```python
from build123d import *

# Parameters (mm, degrees)
F1_DEPTH  = 7.5
F2_DEPTH  = 1.5
F3_DEPTH  = 2
F5_DEPTH  = 45
F6_DEPTH  = 45
F7_W      = 9.5182569801
F7_H      = 1
F8_DEPTH  = 0.5
F9_W      = 12.8092049275
F9_H      = 1
F10_DEPTH = 0.5
F11_R     = 0.49999
F12_R     = 0.49999
F13_W     = 30
F13_H     = 7.6395883262
F14_DEPTH = 11.5
F16_DEPTH = 12.5


# Not quite as in the source:
# - a fillet or chamfer is up to 0.001 mm smaller than in the source, because OpenCascade refuses the exact size


with BuildPart() as f1:
    # F0 (on Front) → F1 (new body)
    with BuildSketch(Plane.XZ):
        with BuildLine():
            Line((-20.75, -40.25), (20.75, -40.25))
            Line((20.75, -40.25), (20.75, -22.75))
            Line((20.75, -22.75), (-9.25, -22.75))
            Line((-9.25, -22.75), (-9.25, 5.25))
            Line((-9.25, 5.25), (20.75, 5.25))
            Line((20.75, 5.25), (20.75, 40.25))
            Line((20.75, 40.25), (-20.75, 40.25))
            Line((-20.75, 40.25), (-20.75, 12.4785664195))
            Line((-20.75, 12.4785664195), (-12.9531003366, 17.9380143384))
            ThreePointArc((-12.9531003366, 17.9380143384), (-2.707082866, 36.9857818255), (14, 23.25))
            ThreePointArc((14, 23.25), (5.1184768061, 10.2192212364), (-10.2573135979, 13.7217515905))
            Line((-10.2573135979, 13.7217515905), (-20.75, 6.3746934757))
            Line((-20.75, 6.3746934757), (-20.75, -40.25))
        make_face()
    extrude(amount=F1_DEPTH)

    # F0 (on Front) → F2 (join)
    with BuildSketch(Plane.XZ):
        with BuildLine():
            ThreePointArc((-12.9531003366, 17.9380143384), (-11.7951280893, 15.7084515279), (-10.2573135979, 13.7217515905))
            Line((-10.2573135979, 13.7217515905), (-6.7277993643, 16.1931440631))
            ThreePointArc((-6.7277993643, 16.1931440631), (-8.3148780488, 18.158310395), (-9.3438531565, 20.4652364212))
            Line((-9.3438531565, 20.4652364212), (-12.9531003366, 17.9380143384))
        make_face()
        with BuildLine():
            Line((-6.7277993643, 16.1931440631), (-10.2573135979, 13.7217515905))
            ThreePointArc((-10.2573135979, 13.7217515905), (5.1184768061, 10.2192212364), (14, 23.25))
            ThreePointArc((14, 23.25), (-2.707082866, 36.9857818255), (-12.9531003366, 17.9380143384))
            Line((-12.9531003366, 17.9380143384), (-9.3438531565, 20.4652364212))
            ThreePointArc((-9.3438531565, 20.4652364212), (-1.4071125975, 32.8979290077), (9.75, 23.25))
            ThreePointArc((9.75, 23.25), (3.8383887374, 14.2873401325), (-6.7277993643, 16.1931440631))
        make_face()
    extrude(amount=F2_DEPTH)

    # F0 (on Front) → F3 (join)
    with BuildSketch(Plane.XZ):
        with BuildLine():
            Line((-20.75, 12.4785664195), (-20.75, 6.3746934757))
            Line((-20.75, 6.3746934757), (-10.2573135979, 13.7217515905))
            ThreePointArc((-10.2573135979, 13.7217515905), (-11.7951280893, 15.7084515279), (-12.9531003366, 17.9380143384))
            Line((-12.9531003366, 17.9380143384), (-20.75, 12.4785664195))
        make_face()
    extrude(amount=F3_DEPTH)

    # F4 (on face) → F5 (cut)
    with BuildSketch(Plane.YZ.offset(20.75)):
        Polygon((-6.4365309663, -40.25), (0, -40.25), (0, -38.5253367255), align=None)
    extrude(amount=-F5_DEPTH, mode=Mode.SUBTRACT)

    # F4 (on face) → F6 (cut)
    with BuildSketch(Plane.YZ.offset(20.75)):
        Polygon((-5.7670628594, -38.0000642006), (0, -36.4547843647), (0, -35.5230358023), (-6, -37.1307309569), align=None)
    extrude(amount=-F6_DEPTH, mode=Mode.SUBTRACT)

    # F7 (on face) → F8 (join)
    with BuildSketch(Plane(origin=(-12.6895494042, 0, 18.122554688), x_dir=(0.8191520443, 0, 0.5735764364), z_dir=(0.5735764364, 0, -0.8191520443))):
        with Locations((-5.0808647713, 7)):
            Rectangle(F7_W, F7_H)
    extrude(amount=F8_DEPTH)

    # F9 (on face) → F10 (join)
    with BuildSketch(Plane(origin=(-9.8216672224, 0, 14.0267944666), x_dir=(0.8191520443, 0, 0.5735764364), z_dir=(-0.5735764364, 0, 0.8191520443))):
        with Locations((-6.9364284886, -7)):
            Rectangle(F9_W, F9_H)
    extrude(amount=F10_DEPTH)

    # F11 (radius 0.5 in the source; OpenCascade refuses exactly that, so slightly less here)
    f11_edges = [f1.edges().sort_by_distance(p)[0] for p in [
        (-20.463212, -7, 12.06899),
        (-16.564762, -6.5, 14.798714),
        (-12.666312, -7, 17.528438),
        (-16.564762, -7.5, 14.798714),
    ]]
    fillet(f11_edges, radius=F11_R)

    # F12 (radius 0.5 in the source; OpenCascade refuses exactly that, so slightly less here)
    f12_edges = [f1.edges().sort_by_distance(p)[0] for p in [
        (-15.790445, -6.5, 10.457799),
        (-21.036788, -7, 6.784269),
        (-15.790445, -7.5, 10.457799),
        (-10.544102, -7, 14.131328),
    ]]
    fillet(f12_edges, radius=F12_R)

    # F13 (on face) → F14 (join)
    with BuildSketch(Plane(origin=(0, 0, 0), x_dir=(-1, 0, 0), z_dir=(0, 1, 0))):
        with Locations((-5.75, -26.5697941631)):
            Rectangle(F13_W, F13_H)
    extrude(amount=-F14_DEPTH)

    # F15 (on face) → F16 (cut, symmetric)
    with BuildSketch(Plane(origin=(0, 0, -30.3895883262), x_dir=(1, 0, 0), z_dir=(0, 0, -1))):
        Polygon((-9.25, 11.5), (20.75, 9.5), (20.75, 11.5), align=None)
    extrude(amount=F16_DEPTH, both=True, mode=Mode.SUBTRACT)


solid = f1.part
```
Source: CAD feature listing. Evaluate the final solid. Frame: model axes, mm. A direction names the side the tool comes from. Coordinates: 2 decimals unless noted, no trailing zeros. Loops run counter-clockwise (first coordinate to the right, second up) from the corner with the lowest first, then second, coordinate; pieces in that order, holes last. Notation, with made-up numbers: M 68.25,25.25 L 112.25,25.25 A22 cw 112.25,52.25 Z; hole C 8,-16.75 d9. An arc over 180 degrees is marked long. Use a Markdown table: item, result. Add a question column.
Q1. Draft query along Y for faces 1 (the flat face through (0.291, -2.924, -37.238)), 2 (the flat face through (20.75, -4, 23)), 3 (the flat face through (0.291, -2.958, -36.316)), 4 (the flat face through (0, 0, -37)). Return one class per face: pulls with the +Y half, pulls with the -Y half, needs draft (parallel to the pull), parting line crosses it, or undercut.
Q2. Access query for faces 5 (the flat face through (-5, 0, 11)), 6 (the flat face through (6, -6, -22.75)), 7 (the flat face through (-10, -1.5, 20)), 8 (the flat face through (-17, -2, 12)). Directions: +Z, -Z, +X, -X, +Y, -Y. A direction counts if a zero-diameter tool reaches every point of the face in a straight line with its end or side. Return the directions, or none.
Q3. First-contact query: pin 1 (1.5 mm diameter, centred on x = -1, y = -9, fed in from +Z); pin 2 (2 mm diameter, centred on y = -5.5, z = -4.5, fed in from -X); pin 3 (4 mm diameter, centred on x = 1, y = -3, fed in from -Z). Flat tips, straight axial feed; report the tip coordinate or a pass-through.
Q4. Section query B-B, the plane z = 19. Return loops of the section in (x, y).
Q5. Section query D-D, the plane y = -4.25. Return loops of the section in (x, z), and give its area (3 significant figures).
Q6. Section query C-C, the plane x = 6.5. Return loops of the section in (y, z).
Q7. Section query A-A, the plane y = -0.75. Return loops of the section in (x, z).
Q8. Material intervals for L1, parallel to X at y = -1.1, z = 23.25; L2, parallel to X at y = -3.8, z = 23.25; L3, parallel to Z at x = 9, y = -4, sorted ascending.
Result:
| question | item | result |
|---|---|---|
| 1 | face 1 | undercut |
| 1 | face 2 | needs draft |
| 1 | face 3 | undercut |
| 1 | face 4 | pulls with the +Y half |
| 2 | face 5 | +Z, -Z, +X, -X, +Y |
| 2 | face 6 | +X, +Y, -Y |
| 2 | face 7 | -Y |
| 2 | face 8 | none |
| 3 | pin 1 | stops at z = -22.75 |
| 3 | pin 2 | stops at x = -20.75 |
| 3 | pin 3 | stops at z = -39.87 |
| 4 | outline | M -20.75,-7.5 L -13.34,-7.5 L -13.34,-1.5 L -8.77,-1.5 L -8.77,0 L -20.75,0 Z; M 8.77,-1.5 L 13.34,-1.5 L 13.34,-7.5 L 20.75,-7.5 L 20.75,0 L 8.77,0 Z |
| 5 | outline | M -20.75,-39.66 L 20.75,-39.66 L 20.75,-37.59 L -20.75,-37.59 Z; M -20.75,-36.66 L 20.75,-36.66 L 20.75,-22.75 L -9.25,-22.75 L -9.25,5.25 L 20.75,5.25 L 20.75,40.25 L -20.75,40.25 L -20.75,12.48 L -12.95,17.94 A14 cw long -10.26,13.72 L -20.75,6.37 Z |
| 5 | area | 1,770 mm2 |
| 6 | outline | M -10.45,-30.39 L -7.5,-30.39 L -7.5,-40.25 L -6.44,-40.25 L 0,-38.53 L 0,-36.45 L -5.77,-38 L -6,-37.13 L 0,-35.52 L 0,-22.75 L -10.45,-22.75 Z; M -7.5,5.25 L 0,5.25 L 0,15.98 L -1.5,15.98 L -1.5,10.85 L -7.5,10.85 Z; M -7.5,35.65 L -1.5,35.65 L -1.5,30.52 L 0,30.52 L 0,40.25 L -7.5,40.25 Z |
| 7 | outline | M -20.75,-38.73 L 20.75,-38.73 L 20.75,-36.66 L -20.75,-36.66 Z; M -20.75,-35.72 L 20.75,-35.72 L 20.75,-22.75 L -9.25,-22.75 L -9.25,5.25 L 20.75,5.25 L 20.75,40.25 L -20.75,40.25 Z; hole C 0,23.25 d19.5 |
| 8 | L1 | x = -20.75 to -9.75, 9.75 to 20.75 |
| 8 | L2 | x = -20.75 to -14, 14 to 20.75 |
| 8 | L3 | z = -39.6 to -37.53, -36.59 to -22.75, 5.25 to 12.53, 33.97 to 40.25 |
